The figure shows three views and two pictorial views of one solid part (mm, origin at its lowest corner). Answer the questions. A direction names the side the tool comes from. Coordinates: 2 decimals unless noted, no trailing zeros. Order: outer loops, then holes, each group sorted by start corner. A loop starts at its lowest first (then second) coordinate and runs counter-clockwise, first axis right, second up. Notation, with made-up numbers: (-29, 81) -> (16, 81) arc R12 ccw to (16, 101) -> close; hole circle Ø9 at (84, 4). An arc over 180 degrees is marked (long way). Write item = value, one per line.
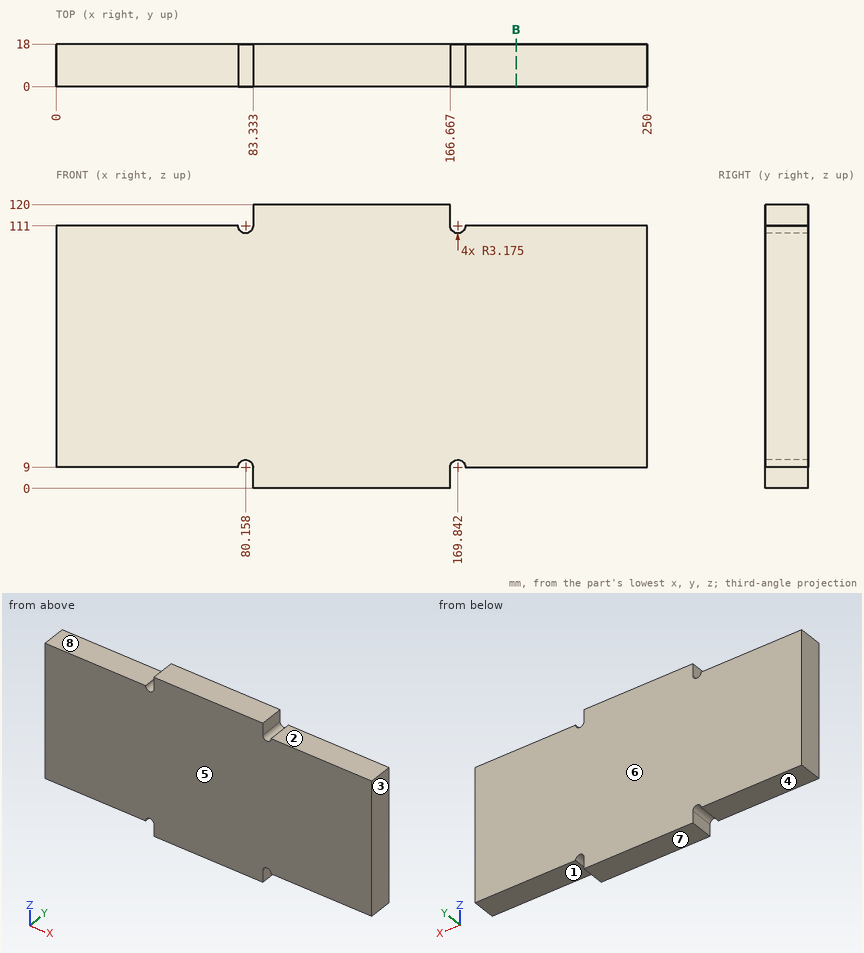
Q1. Section B-B, the plane x = 194.5 is taken. Give the vertices of the cut face in (y, z), plus the area to 3 significant figures.
The answers:
outline = (0, 9) -> (18, 9) -> (18, 111) -> (0, 111) -> close
area = 1,840 mm2
Q2. Find the intervals of material crossed by line 1 along Z through (x, y) = (197, 14); line 2 along X through (y, z) = (6.5, 8); line 3 along Z through (x, y) = (80.5, 13.75), in increasing order.
The answers:
line_1 = 9 to 111
line_2 = 83.33 to 166.67
line_3 = 12.16 to 107.84
Q3. The mould has two halves that part along Z. Classify the marked faces 6, 7 and 8: released by +Z, released by -Z, zero draft, split by the parting line, or undercut.
The answers:
face_6 = zero draft
face_7 = released by -Z
face_8 = released by +Z
Q4. Each of these flat-tipped pins is pushed along its axis until it touches: pin 1 Ø5.5 at (x, y) = (219.5, 13) entering from +Z; pin 2 Ø2.5 at (y, z) = (10.5, 116.5) entering from -X; pin 3 Ø7 at (y, z) = (4.5, 117.5) entering from +X. Where does it stop, or does it pass through?
The answers:
pin_1 = 111
pin_2 = 83.33
pin_3 = 166.67
Q5. A tool of negligible diameter and unlimited length cuts with its end or side. For the marked faces 1, 2, 3, 4 and 5, from which of +Z, -Z, +X, -X, +Y, -Y can it reach the whole face along a straight path? Write none if from no direction.
The answers:
face_1 = -Z, +X, +Y, -Y
face_2 = +Z, +X, +Y, -Y
face_3 = +Z, -Z, +X, +Y, -Y
face_4 = -Z, -X, +Y, -Y
face_5 = +Z, -Z, +X, -X, -Y
